Verification items for the finished model (mm, model axes). A direction names the side the tool comes from. Round coordinates to 2 decimals unless told otherwise and drop trailing zeros. Loops run counter-clockwise (first coordinate to the right, second up) from the corner with the lowest first, then second, coordinate; pieces in that order, holes last. Notation, with made-up numbers: M 13.5,34.25 L 45.5,34.25 A20 cw 45.5,71.25 Z; hole C 34,60.5 d7. An arc over 180 degrees is marked long. One line per item, written item: value.
from build123d import *

# Parameters (mm, degrees)
BOSS_EXTRUDE1_START = 4.0094
SKETCH6_R           = 43.000000106
BOSS_EXTRUDE1_DEPTH = 17.0304
CUT_EXTRUDE1_START  = 4.0094
SKETCH7_R           = 43.000000106
SKETCH7_R_2         = 40.00000001
CUT_EXTRUDE1_DEPTH  = 15.60215


with BuildPart() as part:
    # Sketch5 → Revolve1 (revolve)
    with BuildSketch(Plane.XY):
        Polygon((23.019799782, 10.999999971), (23.019799782, 12.000000003), (18.039799836, 12.000000003), (18.039799836, 31.75), (18.039799836, 35.875000005), (21.039799932, 35.875000005), (21.039799932, 14.999999972), (22.939799942, 14.999999972), (29.909799972, 14.999999972), (29.909799972, 13.99999994), (26.909800003, 10.999999971), align=None)
    revolve(axis=Axis((0, 0, 0), (1, 0, 0)))

    # Sketch6 → Boss-Extrude1 (add)
    with BuildSketch(Plane(origin=(0, 0, 0), x_dir=(0, 0, -1), z_dir=(1, 0, 0)).offset(BOSS_EXTRUDE1_START)):
        with Locations((1.5875, 0)):
            Circle(SKETCH6_R)
        with BuildLine():
            ThreePointArc((-23.952340618, 19.653227004), (-27.928292299, 18.661088308), (-27.323378098, 14.608112886))
            ThreePointArc((-27.323378098, 14.608112886), (-26.399857642, 10.93517908), (-29.65004162, 8.991050256))
            ThreePointArc((-29.65004162, 8.991050256), (-32.943666958, 6.552902785), (-30.833792563, 3.039932389))
            ThreePointArc((-30.833792563, 3.039932389), (-28.575, 0), (-30.833792563, -3.039932389))
            ThreePointArc((-30.833792563, -3.039932389), (-32.943666958, -6.552902785), (-29.65004162, -8.991050256))
            ThreePointArc((-29.65004162, -8.991050256), (-26.399857642, -10.93517908), (-27.323378098, -14.608112886))
            ThreePointArc((-27.323378098, -14.608112886), (-27.928292299, -18.661088308), (-23.952340618, -19.653227004))
            ThreePointArc((-23.952340618, -19.653227004), (-20.205576272, -20.205576272), (-19.653227004, -23.952340618))
            ThreePointArc((-19.653227004, -23.952340618), (-18.661088308, -27.928292299), (-14.608112886, -27.323378098))
            ThreePointArc((-14.608112886, -27.323378098), (-10.93517908, -26.399857642), (-8.991050256, -29.65004162))
            ThreePointArc((-8.991050256, -29.65004162), (-6.552902785, -32.943666958), (-3.039932389, -30.833792563))
            ThreePointArc((-3.039932389, -30.833792563), (0, -28.575), (3.039932389, -30.833792563))
            ThreePointArc((3.039932389, -30.833792563), (6.552902785, -32.943666958), (8.991050256, -29.65004162))
            ThreePointArc((8.991050256, -29.65004162), (10.93517908, -26.399857642), (14.608112886, -27.323378098))
            ThreePointArc((14.608112886, -27.323378098), (18.661088308, -27.928292299), (19.653227004, -23.952340618))
            ThreePointArc((19.653227004, -23.952340618), (20.205576272, -20.205576272), (23.952340618, -19.653227004))
            ThreePointArc((23.952340618, -19.653227004), (27.928292299, -18.661088308), (27.323378098, -14.608112886))
            ThreePointArc((27.323378098, -14.608112886), (26.399857642, -10.93517908), (29.65004162, -8.991050256))
            ThreePointArc((29.65004162, -8.991050256), (32.943666958, -6.552902785), (30.833792563, -3.039932389))
            ThreePointArc((30.833792563, -3.039932389), (28.575, 0), (30.833792563, 3.039932389))
            ThreePointArc((30.833792563, 3.039932389), (32.943666958, 6.552902785), (29.65004162, 8.991050256))
            ThreePointArc((29.65004162, 8.991050256), (26.399857642, 10.93517908), (27.323378098, 14.608112886))
            ThreePointArc((27.323378098, 14.608112886), (27.928292299, 18.661088308), (23.952340618, 19.653227004))
            ThreePointArc((23.952340618, 19.653227004), (20.205576272, 20.205576272), (19.653227004, 23.952340618))
            ThreePointArc((19.653227004, 23.952340618), (18.661088308, 27.928292299), (14.608112886, 27.323378098))
            ThreePointArc((14.608112886, 27.323378098), (10.93517908, 26.399857642), (8.991050256, 29.65004162))
            ThreePointArc((8.991050256, 29.65004162), (6.552902785, 32.943666958), (3.039932389, 30.833792563))
            ThreePointArc((3.039932389, 30.833792563), (0, 28.575), (-3.039932389, 30.833792563))
            ThreePointArc((-3.039932389, 30.833792563), (-6.552902785, 32.943666958), (-8.991050256, 29.65004162))
            ThreePointArc((-8.991050256, 29.65004162), (-10.93517908, 26.399857642), (-14.608112886, 27.323378098))
            ThreePointArc((-14.608112886, 27.323378098), (-18.661088308, 27.928292299), (-19.653227004, 23.952340618))
            ThreePointArc((-19.653227004, 23.952340618), (-20.205576272, 20.205576272), (-23.952340618, 19.653227004))
        make_face(mode=Mode.SUBTRACT)
    extrude(amount=BOSS_EXTRUDE1_DEPTH)

    # Sketch7 → Cut-Extrude1 (cut)
    with BuildSketch(Plane(origin=(0, 0, 0), x_dir=(0, 0, -1), z_dir=(1, 0, 0)).offset(CUT_EXTRUDE1_START)):
        with Locations((1.5875, 0)):
            Circle(SKETCH7_R)
        with Locations((1.5875, 0)):
            Circle(SKETCH7_R_2, mode=Mode.SUBTRACT)
    extrude(amount=CUT_EXTRUDE1_DEPTH, mode=Mode.SUBTRACT)


solid = part.part
(1) Mould release check, pull along Z, two halves, no side actions. Record for faces 3 (the face through (4.009, -12, -28)), 4 (the face through (11.7, 12.01, -39.74)), 5 (the face through (10.926, 0.057, 28.576)): +Z half, -Z half, draft (parallel to the pull), parting line (faces both ways), or undercut.
Completed:
face 3: draft
face 4: parting line
face 5: undercut
(2) Sectioned sample at D-D on y = -25. Enter the section's corners in (x, z), and give its area (3 significant figures).
Completed:
outline: M 4.01,-32.81 L 19.61,-32.81 L 19.61,-36.57 L 21.04,-36.57 L 21.04,33.4 L 19.61,33.4 L 19.61,29.64 L 4.01,29.64 L 4.01,19.99 L 18.04,19.99 L 18.04,-19.99 L 4.01,-19.99 Z
area: 513 mm^2
(3) Sectioned sample at C-C on z = 0. Enter the section's corners in (x, y) (3 decimals).
Completed:
outline: M 4.009,-39.968 L 19.612,-39.968 L 19.612,-42.971 L 21.04,-42.971 L 21.04,-15 L 29.91,-15 L 29.91,-14 L 26.91,-11 L 23.02,-11 L 23.02,-12 L 18.04,-12 L 18.04,-28.575 L 4.009,-28.575 Z; M 4.009,28.575 L 18.04,28.575 L 18.04,12 L 23.02,12 L 23.02,11 L 26.91,11 L 29.91,14 L 29.91,15 L 21.04,15 L 21.04,42.971 L 19.612,42.971 L 19.612,39.968 L 4.009,39.968 Z
(4) Depth check by flat-ended pin: pin 1 Ø10 at (x, y) = (22, -18.5) entering from -Z; pin 2 Ø1.5 at (x, z) = (20, 23) entering from +Y; pin 3 Ø12 at (y, z) = (29.5, -13.5) entering from +X. Enter the tip coordinate at first touch or a pass-through.
Completed:
pin 1: stops at z = -42.38
pin 2: stops at y = 35.79
pin 3: stops at x = 21.04
(5) Tool access check on faces 1 (the face through (25, -12, -9)), 2 (the face through (10.93, 6.61, 32.93)). Record the directions out of +Z, -Z, +X, -X, +Y, -Y that give a thin tool (end or side, any length) a straight path to the whole face; none if there is none.
Completed:
face 1: +X
face 2: -X
(6) Thickness scan on L1, parallel to Z at x = 21.35, y = 0; L2, parallel to X at y = -20, z = -15.5; L3, parallel to Z at x = 24.6, y = 0. Record the ranges inside material, lowest first. Write a range as from..to.
Completed:
L1: z = -15..-12, 12..15
L2: x = 18.04..21.04
L3: z = -15..-11, 11..15
(7) Sectioned sample at A-A on y = 0. Enter the section's corners in (x, z) (1 decimal).
Completed:
outline: M 4,-41.6 L 19.6,-41.6 L 19.6,-44.6 L 21,-44.6 L 21,-15 L 29.9,-15 L 29.9,-14 L 26.9,-11 L 23,-11 L 23,-12 L 18,-12 L 18,-28.6 L 4,-28.6 Z; M 4,28.6 L 18,28.6 L 18,12 L 23,12 L 23,11 L 26.9,11 L 29.9,14 L 29.9,15 L 21,15 L 21,41.4 L 19.6,41.4 L 19.6,38.4 L 4,38.4 Z
